Could you check a few things on this drawing? It's one solid part, dimensions in mm from its lowest x, y, z. A direction names the side the tool comes from. Round coordinates to 2 decimals unless told otherwise and drop trailing zeros. Write each loop counter-clockwise with the first axis right and the second up, starting at its lowest first coordinate (ties: lowest second). Pieces come first, ordered by that corner, then holes. Notation, with made-up numbers: (10, 89) -> (16, 89) arc R16 ccw to (16, 114) -> close; hole circle Ø5 at (-3.75, 86.5). An arc over 180 degrees is marked (long way). Put each result on its own line as item: value. Start each with the question number.
1) I want a section at C-C, the plane z = 1.15. List the corners of the cut face in (x, y) for me, then the cut area to 3 significant figures.
2) Will these pins go through, and if not, where does the flat tip stop? P1, Ø1, axis at x = 4.5, z = 2.5, coming from the +Y side; P2, Ø1, axis at y = 4.5, z = 2.5, coming from the -X side.
3) If I drill on line 1 along Y through (x, z) = (0.5, 0.9); line 2 along Z through (x, y) = (5.5, 2.5); line 3 along Z through (x, y) = (7.5, 5), over which ranges is the centre line in solid material (lowest first)? Write a range as [from, to].
4) Which directions (+Z, -Z, +X, -X, +Y, -Y) give clear straight access to the entire face, cutting with the end or side of a thin tool? Please do the marked faces 1 and 2.
5) I want a section at B-B, the plane z = 1.7. List the corners of the cut face in (x, y) for me.
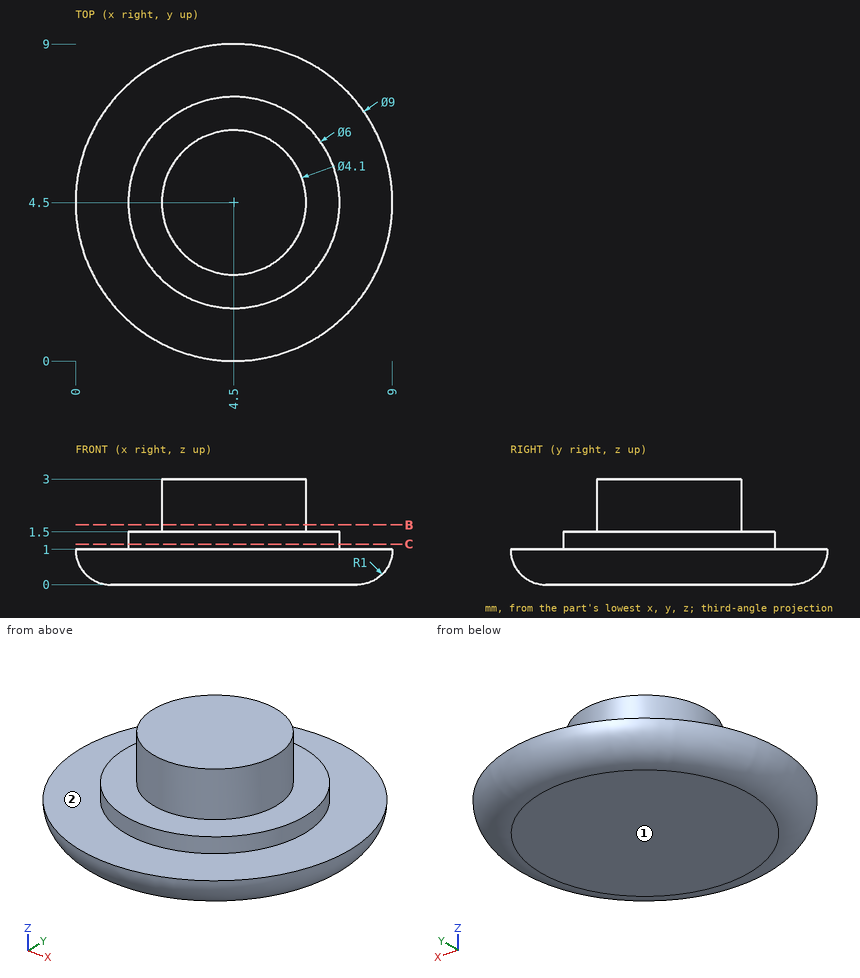
Findings:
1. outline: circle Ø6 at (4.5, 4.5)
1. area: 28.3 mm2
2. P1: stops at y = 6.55
2. P2: stops at x = 2.45
3. line 1: y = [2.45, 6.55]
3. line 2: z = [0, 1.5]
3. line 3: z = [0, 1]
4. face 1: -Z, +X, -X, +Y, -Y
4. face 2: +Z
5. outline: circle Ø4.1 at (4.5, 4.5)
